from build123d import *

# Parameters (mm, degrees)
BOSS_EXTRU_1_DEPTH      = 15
BOSS_EXTRU_2_DEPTH      = 5
ENL_V_MAT_EXTRU_1_DEPTH = 20
ESQUISSE4_R             = 2.9
ESQUISSE4_R_2           = 1.6
ENL_V_MAT_EXTRU_2_DEPTH = 12
ENL_V_MAT_EXTRU_3_DEPTH = 12
ESQUISSE7_R             = 1.5
ENL_V_MAT_EXTRU_5_DEPTH = 15


with BuildPart() as part:
    # Esquisse1 → Boss.-Extru.1 (new body)
    with BuildSketch(Plane.XY):
        Polygon((0, 20), (20, 0), (20, 20), align=None)
        with BuildLine():
            Line((20, 17), (20, 0))
            Line((20, 0), (40, 0))
            Line((40, 0), (40, 17))
            Line((40, 17), (35, 17))
            ThreePointArc((35, 17), (30, 12), (25, 17))
            Line((25, 17), (20, 17))
        make_face()
        Polygon((40, 0), (40, 20), (60, 20), align=None)
    extrude(amount=BOSS_EXTRU_1_DEPTH)

    # Esquisse3 → Boss.-Extru.2 (add)
    with BuildSketch(Plane.XY.offset(15)):
        with BuildLine():
            Line((25, 17), (35, 17))
            ThreePointArc((35, 17), (30, 12), (25, 17))
        make_face()
        with BuildLine():
            Line((20, 20), (0, 20))
            Line((0, 20), (20, 0))
            Line((20, 0), (40, 0))
            Line((40, 0), (60, 20))
            Line((60, 20), (40, 20))
            Line((40, 20), (40, 17))
            Line((40, 17), (35, 17))
            ThreePointArc((35, 17), (30, 12), (25, 17))
            Line((25, 17), (20, 17))
            Line((20, 17), (20, 20))
        make_face()
    extrude(amount=BOSS_EXTRU_2_DEPTH)

    # Esquisse2 → Enlèv. mat.-Extru.1 (cut)
    with BuildSketch(Plane(origin=(0, 20, 0), x_dir=(1, 0, 0), z_dir=(0, 1, 0))):
        with BuildLine():
            ThreePointArc((31.6, -10), (31.13137085, -8.86862915), (30, -8.4))
            Line((30, -8.4), (30, -10))
            Line((30, -10), (31.6, -10))
        make_face()
        with BuildLine():
            Line((30, -10), (30, -8.4))
            ThreePointArc((30, -8.4), (28.86862915, -11.13137085), (31.6, -10))
            Line((31.6, -10), (30, -10))
        make_face()
    extrude(amount=-ENL_V_MAT_EXTRU_1_DEPTH, mode=Mode.SUBTRACT)

    # Esquisse4 → Enlèv. mat.-Extru.2 (cut)
    with BuildSketch(Plane(origin=(0, 20, 0), x_dir=(1, 0, 0), z_dir=(0, 1, 0))):
        with Locations((30, -10)):
            Circle(ESQUISSE4_R)
        with Locations((30, -10)):
            Circle(ESQUISSE4_R_2, mode=Mode.SUBTRACT)
    extrude(amount=-ENL_V_MAT_EXTRU_2_DEPTH, mode=Mode.SUBTRACT)

    # Esquisse5 → Enlèv. mat.-Extru.3 (cut)
    with BuildSketch(Plane(origin=(0, 20, 0), x_dir=(1, 0, 0), z_dir=(0, 1, 0))):
        with BuildLine():
            ThreePointArc((51.5, -10), (51.385819299, -9.425974851), (51.060660172, -8.939339828))
            Line((51.060660172, -8.939339828), (50, -10))
            Line((50, -10), (51.060660172, -11.060660172))
            ThreePointArc((51.060660172, -11.060660172), (51.385819299, -10.574025149), (51.5, -10))
        make_face()
        with BuildLine():
            Line((50, -10), (51.060660172, -8.939339828))
            ThreePointArc((51.060660172, -8.939339828), (50, -8.5), (48.939339828, -8.939339828))
            Line((48.939339828, -8.939339828), (50, -10))
        make_face()
        with BuildLine():
            Line((50, -10), (48.939339828, -8.939339828))
            ThreePointArc((48.939339828, -8.939339828), (48.5, -10), (48.939339828, -11.060660172))
            Line((48.939339828, -11.060660172), (50, -10))
        make_face()
        with BuildLine():
            ThreePointArc((48.939339828, -11.060660172), (50, -11.5), (51.060660172, -11.060660172))
            Line((51.060660172, -11.060660172), (50, -10))
            Line((50, -10), (48.939339828, -11.060660172))
        make_face()
        with BuildLine():
            ThreePointArc((11.5, -10), (11.385819299, -9.425974851), (11.060660172, -8.939339828))
            Line((11.060660172, -8.939339828), (10, -10))
            Line((10, -10), (11.060660172, -11.060660172))
            ThreePointArc((11.060660172, -11.060660172), (11.385819299, -10.574025149), (11.5, -10))
        make_face()
        with BuildLine():
            Line((10, -10), (11.060660172, -8.939339828))
            ThreePointArc((11.060660172, -8.939339828), (10, -8.5), (8.939339828, -8.939339828))
            Line((8.939339828, -8.939339828), (10, -10))
        make_face()
        with BuildLine():
            Line((10, -10), (8.939339828, -8.939339828))
            ThreePointArc((8.939339828, -8.939339828), (8.5, -10), (8.939339828, -11.060660172))
            Line((8.939339828, -11.060660172), (10, -10))
        make_face()
        with BuildLine():
            ThreePointArc((8.939339828, -11.060660172), (10, -11.5), (11.060660172, -11.060660172))
            Line((11.060660172, -11.060660172), (10, -10))
            Line((10, -10), (8.939339828, -11.060660172))
        make_face()
    extrude(amount=-ENL_V_MAT_EXTRU_3_DEPTH, mode=Mode.SUBTRACT)

    # Esquisse7 → Enlèv. mat.-Extru.5 (cut)
    with BuildSketch(Plane.XZ):
        Polygon((10, 6.882308546), (12.7, 8.441154273), (12.7, 11.558845727), (10, 13.117691454), (7.3, 11.558845727), (7.3, 8.441154273), align=None)
        with Locations((10, 10)):
            Circle(ESQUISSE7_R, mode=Mode.SUBTRACT)
        Polygon((50, 6.882308546), (52.7, 8.441154273), (52.7, 11.558845727), (50, 13.117691454), (47.3, 11.558845727), (47.3, 8.441154273), align=None)
        with Locations((50, 10)):
            Circle(ESQUISSE7_R, mode=Mode.SUBTRACT)
    extrude(amount=-ENL_V_MAT_EXTRU_5_DEPTH, mode=Mode.SUBTRACT)


solid = part.part
Source: CAD feature listing. Evaluate the final solid. Frame: model axes, mm. A direction names the side the tool comes from. Coordinates: 2 decimals unless noted, no trailing zeros. Order: outer loops, then holes, each group sorted by start corner. A loop starts at its lowest first (then second) coordinate and runs counter-clockwise, first axis right, second up.
Item 1: Cut plane A-A (y = 17.75). Return loops of the section in (x, z).
Output values:
outline: (2.25, 0) - (20, 0) - (20, 20) - (2.25, 20) - close; (40, 0) - (57.75, 0) - (57.75, 20) - (40, 20) - close; hole circle Ø3 at (10, 10); hole circle Ø3 at (50, 10)
Item 2: Set-up query: faces 4 (the face through (32.766, 10.498, 9.129)), 5 (the face through (48.8, 15, 8.7)), 6 (the face through (30, 17, 17)). Return all of +Z, -Z, +X, -X, +Y, -Y with unobstructed straight access to the full face (end or side cutting, diameter ignored); none if empty.
Output values:
face 4: +Y
face 5: -Y
face 6: +Z, -Z, +Y
Item 3: Cut plane B-B (y = 5). Return loops of the section in (x, z).
Output values:
outline: (15, 0) - (45, 0) - (45, 20) - (15, 20) - close; hole circle Ø3.2 at (30, 10)
Item 4: Cut plane D-D (x = 18). Return loops of the section in (y, z), plus the area to 3 significant figures.
Output values:
outline: (2, 0) - (20, 0) - (20, 20) - (2, 20) - close
area: 360 mm2
Item 5: Cut plane C-C (z = 18). Return loops of the section in (x, y).
Output values:
outline: (0, 20) - (20, 0) - (40, 0) - (60, 20) - (40, 20) - (40, 17) - (20, 17) - (20, 20) - close
Item 6: Pull-direction query (Z, two-part tool) for faces 1 (the face through (11.369, 11.952, 12.327)), 2 (the face through (20, 18, 10)), 3 (the face through (30, 10, 0)); classes: pulls with the +Z half, pulls with the -Z half, needs draft (parallel to the pull), parting line crosses it, or undercut.
Output values:
face 1: undercut
face 2: needs draft
face 3: pulls with the -Z half
Item 7: First-contact query: P1, Ø1.5, axis at y = 18.5, z = 13, coming from the -X side; P2, Ø1.5, axis at x = 13, z = 16.5, coming from the -Y side; P3, Ø0.9, axis at y = 18.5, z = 13.5, coming from the +X side. Flat tips, straight axial feed; report the tip coordinate or a pass-through.
Output values:
P1: stops at x = 0.75
P2: stops at y = 6.25
P3: stops at x = 58.95
Item 8: Material intervals for line 1 (X direction, y = 10.2, z = 10); line 2 (Z direction, x = 30, y = 10.9); line 3 (Z direction, x = 30, y = 1.5), sorted ascending.
Output values:
line 1: x = 12.7 to 27.1, 32.9 to 47.3
line 2: z = 0 to 7.1, 12.9 to 20
line 3: z = 0 to 8.4, 11.6 to 20
